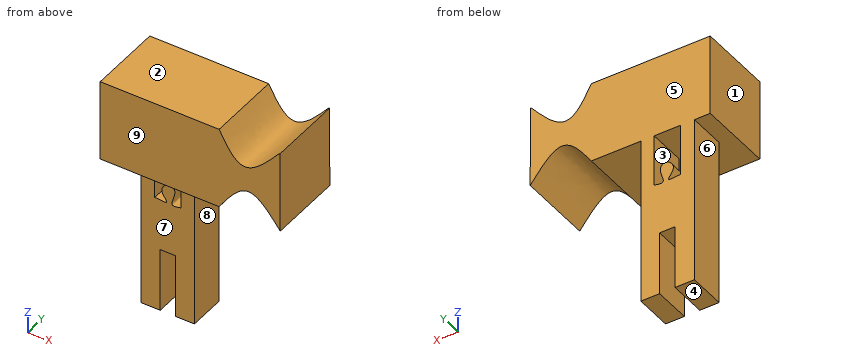
```python
from build123d import *

# Parameters (mm, degrees)
F1_DEPTH = 25.4
F3_DEPTH = 12.7


with BuildPart() as f1:
    # F0 (on Front) → F1 (new body)
    with BuildSketch(Plane.XZ):
        with BuildLine():
            Line((-5.9723113663, 45.0293272734), (-46.1669079959, 45.0293272734))
            Line((-46.1669079959, 45.0293272734), (-46.1669079959, 17.5377372652))
            Line((-46.1669079959, 17.5377372652), (-5.9723113663, 17.5377372652))
            add(Edge.make_bspline(
                [(-5.9723113663, 17.5377372652), (-2.7421037419, 22.2388113669), (3.7997517849, 31.7594834628), (11.0324224964, 22.3175007577), (14.6937780082, 17.5377372652)],
                knots=[0, 0, 0, 0, 0.4937754451, 1, 1, 1, 1], degree=3))
            Line((14.6937780082, 17.5377372652), (14.6510465513, 45.0568711834))
            add(Edge.make_bspline(
                [(-5.9723113663, 45.0293272734), (-3.1039018596, 39.7353803072), (2.6906778005, 29.0408831168), (14.035828108, 45.0860466111), (14.6176635276, 45.0721417685), (14.6510465513, 45.0568711834)],
                knots=[0, 0, 0, 0, 0.4677545083, 0.944928105, 0.9824927302, 0.9824927302, 0.9824927302, 0.9824927302], degree=3))
        make_face()
    extrude(amount=F1_DEPTH)

    # F2 (on Front) → F3 (join)
    with BuildSketch(Plane.XZ):
        with BuildLine():
            Line((-40.8112728043, -17.1658259542), (-40.8112728043, -39.3341283589))
            Line((-40.8112728043, -39.3341283589), (-34.2571637339, -39.3341283589))
            Line((-34.2571637339, -39.3341283589), (-34.2571637339, -17.7441283589))
            Line((-34.2571637339, -17.7441283589), (-29.0524326225, -17.7441283589))
            Line((-29.0524326225, -17.7441283589), (-29.0524326225, -39.3341283589))
            Line((-29.0524326225, -39.3341283589), (-22.7024326225, -39.3341283589))
            Line((-22.7024326225, -39.3341283589), (-22.7024326225, -17.1658259542))
            Line((-22.7024326225, -17.1658259542), (-22.7024326225, 0))
            Line((-22.7024326225, 0), (-22.7024326225, 17.9169308394))
            Line((-22.7024326225, 17.9169308394), (-27.2071920335, 17.9169308394))
            Line((-27.2071920335, 17.9169308394), (-27.2071920335, 0))
            add(Edge.make_bspline(
                [(-27.2071920335, 0), (-28.5825818847, -0.3177946326), (-31.6773810864, -1.0328723065), (-28.2469905577, 4.7548163588), (-31.0048564618, 7.3974553181), (-33.9624208414, 4.7018522539), (-33.6773839228, 2.2731173072), (-30.9591203554, -0.6389776746), (-34.9429871553, 0.1082431292), (-35.7740289914, 0.0317036785), (-36.1182577908, 0)],
                knots=[0, 0, 0, 0, 0.131934451, 0.2968690174, 0.4178502166, 0.5514286485, 0.6705283065, 0.7893202312, 0.9127335825, 1, 1, 1, 1], degree=3))
            Line((-36.1182577908, 0), (-36.1182577908, 17.9169308394))
            Line((-36.1182577908, 17.9169308394), (-40.8112728043, 17.9169308394))
            Line((-40.8112728043, 17.9169308394), (-40.8112728043, 0))
            Line((-40.8112728043, 0), (-40.8112728043, -17.1658259542))
        make_face()
    extrude(amount=F3_DEPTH)


solid = f1.part
```
The listing builds one solid part. Answer for the finished solid, in the listing's coordinates (mm). Face numbers are marked on the shaded views. A direction names the side the tool comes from. Give positions to 0.01 mm unless a question says otherwise; leave off trailing zeros. Order: outer loops, then holes, each group sorted by start corner. A loop starts at its lowest first (then second) coordinate and runs counter-clockwise, first axis right, second up.
Item 1: Which of the six approach directions +Z, -Z, +X, -X, +Y, -Y give full straight-line access (tool end or side, diameter ignored) to the marked faces 5, 6, 7, 8 and 9?
From the geometry:
face 5: +Z, -Z, +X, -X, +Y
face 6: -Z, -X, +Y, -Y
face 7: -Z, +X, -X, -Y
face 8: -Z, +X, +Y, -Y
face 9: +Z, -Z, +X, -X, -Y
Item 2: The part is cut by section B-B, the plane x = -24.5. Give the vertices of the cut face in (y, z), and give its area (3 significant figures).
From the geometry:
outline: (-25.4, 17.54) - (-12.7, 17.54) - (-12.7, -39.33) - (0, -39.33) - (0, 45.03) - (-25.4, 45.03) - close
area: 1,420 mm2
Item 3: Find the intervals of material crossed by probe 1 along X at (y, z) = (-12, -23); probe 2 along Z at (x, y) = (-25, -5); probe 3 along X at (y, z) = (-12, 1), in increasing order.
From the geometry:
probe 1: x = -40.81 to -34.26, -29.05 to -22.7
probe 2: z = -39.33 to 45.03
probe 3: x = -40.81 to -36.12, -32.49 to -30.2, -27.21 to -22.7
Item 4: The part is cut by section A-A, the plane z = -24. Give the vertices of the cut face in (x, y), and give its area (3 significant figures).
From the geometry:
outline: (-40.81, -12.7) - (-34.26, -12.7) - (-34.26, 0) - (-40.81, 0) - close; (-29.05, -12.7) - (-22.7, -12.7) - (-22.7, 0) - (-29.05, 0) - close
area: 164 mm2
Item 5: Given pin 1 Ø4 at (x, y) = (-6, -15.5) entering from +Z; pin 2 Ø12 at (y, z) = (-18.5, 0) entering from +X; pin 3 Ø5.5 at (x, z) = (-35.5, 2) entering from -Y, each flat-ended and moving along its own axis, determine where each tip first touches the part or whether it passes through.
From the geometry:
pin 1: stops at z = 45.03
pin 2: stops at x = -22.7
pin 3: stops at y = -12.7
Item 6: The part is cut by section C-C, the plane z = 4.5. Count the separate pieces of the cut face and the enclosed holes in it, and give its area (3 significant figures).
From the geometry:
separate pieces: 3
enclosed holes: 0
area: 171 mm2
Item 7: For a pull along Z with two mould halves and no side action, classify the marked faces 1, 2, 3 and 4 as pulls with the +Z half, pulls with the -Z half, needs draft (parallel to the pull), parting line crosses it, or undercut.
From the geometry:
face 1: needs draft
face 2: pulls with the +Z half
face 3: undercut
face 4: pulls with the -Z half
Item 8: The part is cut by section D-D, the plane z = -14. Give the vertices of the cut face in (x, y), and give its area (3 significant figures).
From the geometry:
outline: (-40.81, -12.7) - (-22.7, -12.7) - (-22.7, 0) - (-40.81, 0) - close
area: 230 mm2
